```python
from build123d import *

# Parameters (mm, degrees)
SALIENTE_EXTRUIR1_DEPTH = 250
REDONDEO1_R             = 1.5
REDONDEO2_R             = 0.5
CORTAR_EXTRUIR1_DEPTH   = 251.399680511


with BuildPart() as part:
    # Croquis1 → Saliente-Extruir1 (new body)
    with BuildSketch(Plane.XY):
        Polygon((3, -4.5), (5.7413765, -7.2413765), (5.7413765, -8.5), (3, -8.5), (3, -10), (10, -10), (10, -3), (8.5, -3), (8.5, -5.7413765), (7.2413765, -5.7413765), (4.5, -3), (4.5, 3), (7.2413765, 5.7413765), (8.5, 5.7413765), (8.5, 3), (10, 3), (10, 10), (3, 10), (3, 8.5), (5.7413765, 8.5), (5.7413765, 7.2413765), (3, 4.5), (-3, 4.5), (-5.7413765, 7.2413765), (-5.7413765, 8.5), (-3, 8.5), (-3, 10), (-10, 10), (-10, 3), (-8.5, 3), (-8.5, 5.7413765), (-7.2413765, 5.7413765), (-4.5, 3), (-4.5, -3), (-7.2413765, -5.7413765), (-8.5, -5.7413765), (-8.5, -3), (-10, -3), (-10, -10), (-3, -10), (-3, -8.5), (-5.7413765, -8.5), (-5.7413765, -7.2413765), (-3, -4.5), align=None)
    extrude(amount=SALIENTE_EXTRUIR1_DEPTH)

    # Redondeo1
    redondeo1_edges = [part.edges().sort_by_distance(p)[0] for p in [
        (10, -10, 125),
        (-10, -10, 125),
        (-10, 10, 125),
        (10, 10, 125),
    ]]
    fillet(redondeo1_edges, radius=REDONDEO1_R)

    # Redondeo2
    redondeo2_edges = [part.edges().sort_by_distance(p)[0] for p in [
        (-5.7413765, -8.5, 125),
        (-8.5, -5.7413765, 125),
        (-8.5, 5.7413765, 125),
        (-5.7413765, 8.5, 125),
        (5.7413765, 8.5, 125),
        (8.5, 5.7413765, 125),
        (8.5, -5.7413765, 125),
    ]]
    fillet(redondeo2_edges, radius=REDONDEO2_R)

    # Croquis2 → Cortar-Extruir1 (cut, through all)
    with BuildSketch(Plane(origin=(0, 0, 0), x_dir=(-1, 0, 0), z_dir=(0, 0, -1))):
        with BuildLine():
            Line((-1.340498607, 2.401158779), (-1.870828693, 2.931488865))
            Line((-1.870828693, 2.931488865), (-2.931488865, 1.870828693))
            Line((-2.931488865, 1.870828693), (-2.401158779, 1.340498607))
            ThreePointArc((-2.401158779, 1.340498607), (-2.75, 0), (-2.401158779, -1.340498607))
            Line((-2.401158779, -1.340498607), (-2.931488865, -1.870828693))
            Line((-2.931488865, -1.870828693), (-1.870828693, -2.931488865))
            Line((-1.870828693, -2.931488865), (-1.340498607, -2.401158779))
            ThreePointArc((-1.340498607, -2.401158779), (0, -2.75), (1.340498607, -2.401158779))
            Line((1.340498607, -2.401158779), (1.870828693, -2.931488865))
            Line((1.870828693, -2.931488865), (2.931488865, -1.870828693))
            Line((2.931488865, -1.870828693), (2.401158779, -1.340498607))
            ThreePointArc((2.401158779, -1.340498607), (2.75, 0), (2.401158779, 1.340498607))
            Line((2.401158779, 1.340498607), (2.931488865, 1.870828693))
            Line((2.931488865, 1.870828693), (1.870828693, 2.931488865))
            Line((1.870828693, 2.931488865), (1.340498607, 2.401158779))
            ThreePointArc((1.340498607, 2.401158779), (0, 2.75), (-1.340498607, 2.401158779))
        make_face()
    extrude(amount=-CORTAR_EXTRUIR1_DEPTH, mode=Mode.SUBTRACT)


solid = part.part
```
Verification items for the finished model (mm, model axes). A direction names the side the tool comes from. Coordinates: 2 decimals unless noted, no trailing zeros. Put each result on its own line as item: value.
1. Thickness scan on line 1 (Y direction, x = 4.25, z = 31.5); line 2 (X direction, y = -8.75, z = 33.5). Record the ranges inside material, lowest first.
Result set:
line 1: y = -10 to -8.5, -5.75 to 5.75, 8.5 to 10
line 2: x = -9.98 to -3, 3 to 9.98
2. Gauge pin test, flat ends, axial feed: P1, Ø1.8, axis at y = 1, z = 129, coming from the -X side; P2, Ø1.2, axis at x = 9.5, z = 108.5, coming from the -Y side; P3, Ø0.8, axis at x = -9, z = 72, coming from the +Y side. Record the tip position at first contact, or that the pin passes through.
Result set:
P1: stops at x = -4.5
P2: stops at y = -9.95
P3: stops at y = 10
3. Tool access check on faces 4 (the face through (4.5, 0, 123)), 5 (the face through (-4.5, 0, 123)), 6 (the face through (0, -4, 0)), 7 (the face through (0, -4.5, 123)). Record the directions out of +Z, -Z, +X, -X, +Y, -Y that give a thin tool (end or side, any length) a straight path to the whole face; none if there is none.
Result set:
face 4: +Z, -Z, +X
face 5: +Z, -Z, -X
face 6: -Z, +X, -X, +Y, -Y
face 7: +Z, -Z, -Y
4. Mould release check, pull along X, two halves, no side actions. Record for faces 1 (the face through (0, 4.5, 123)), 2 (the face through (-6, 10, 123)), 3 (the face through (10, -6, 123)): pulls with the +X half, pulls with the -X half, needs draft (parallel to the pull), parting line crosses it, or undercut.
Result set:
face 1: undercut
face 2: needs draft
face 3: pulls with the +X half
